The model under review builds one solid part; all positions refer to its coordinate system, in mm. A direction names the side the tool comes from. Give positions to 0.01 mm unless a question says otherwise; leave off trailing zeros. Order: outer loops, then holes, each group sorted by start corner. A loop starts at its lowest first (then second) coordinate and runs counter-clockwise, first axis right, second up. Notation, with made-up numbers: (56, 1) -> (73, 1) arc R12 ccw to (73, 6) -> close; hole circle Ø11 at (-39.5, 36). An arc over 180 degrees is marked (long way). Use one line per item in the form item = value.
```python
from build123d import *

# Parameters (mm, degrees)
SKETCH1_W           = 120
SKETCH1_H           = 75
BOSS_EXTRUDE1_DEPTH = 3
CHAMFER1_SIZE       = 6
SKETCH2_W           = 109.5
SKETCH2_H           = 64.5
BOSS_EXTRUDE2_DEPTH = 2
CHAMFER2_SIZE       = 7
SKETCH3_R           = 1.5
CUT_EXTRUDE1_DEPTH  = 5
SKETCH4_W           = 5.25
SKETCH4_H           = 9.5
SKETCH4_H_2         = 14.5
BOSS_EXTRUDE3_DEPTH = 5


with BuildPart() as part:
    # Sketch1 → Boss-Extrude1 (new body)
    with BuildSketch(Plane(origin=(0, 0, 0), x_dir=(1, 0, 0), z_dir=(0, 1, 0))):
        Rectangle(SKETCH1_W, SKETCH1_H)
    extrude(amount=BOSS_EXTRUDE1_DEPTH)

    # Chamfer1
    chamfer1_edges = [part.edges().sort_by_distance(p)[0] for p in [
        (60, 1.5, 37.5),
        (-60, 1.5, 37.5),
        (-60, 1.5, -37.5),
        (60, 1.5, -37.5),
    ]]
    chamfer(chamfer1_edges, length=CHAMFER1_SIZE)

    # Sketch2 → Boss-Extrude2 (add)
    with BuildSketch(Plane(origin=(0, 3, 0), x_dir=(1, 0, 0), z_dir=(0, 1, 0))):
        Rectangle(SKETCH2_W, SKETCH2_H)
    extrude(amount=BOSS_EXTRUDE2_DEPTH)

    # Chamfer2
    chamfer2_edges = [part.edges().sort_by_distance(p)[0] for p in [
        (54.75, 4, 32.25),
        (54.75, 4, -32.25),
        (-54.75, 4, -32.25),
        (-54.75, 4, 32.25),
    ]]
    chamfer(chamfer2_edges, length=CHAMFER2_SIZE)

    # Sketch3 → Cut-Extrude1 (cut)
    with BuildSketch(Plane(origin=(0, 3, 0), x_dir=(1, 0, 0), z_dir=(0, 1, 0))):
        with Locations(Location((-54.5, -32, 0), (0, 0, 270))):
            Circle(SKETCH3_R)
        with Locations(Location((-54.5, 32, 0), (0, 0, 270))):
            Circle(SKETCH3_R)
        with Locations(Location((54.5, 32, 0), (0, 0, 270))):
            Circle(SKETCH3_R)
        with Locations(Location((54.5, -32, 0), (0, 0, 270))):
            Circle(SKETCH3_R)
    extrude(amount=-CUT_EXTRUDE1_DEPTH, mode=Mode.SUBTRACT)

    # Sketch4 → Boss-Extrude3 (add)
    with BuildSketch(Plane(origin=(0, 3, 0), x_dir=(1, 0, 0), z_dir=(0, 1, 0))):
        with Locations((57.375, 19.5)):
            Rectangle(SKETCH4_W, SKETCH4_H)
        with Locations((57.375, -12)):
            Rectangle(SKETCH4_W, SKETCH4_H_2)
    extrude(amount=BOSS_EXTRUDE3_DEPTH)


solid = part.part
```
1. The part is to be moulded in two halves that separate along Z. For faces 1 (the face through (57, 5, 4.75)), 2 (the face through (54.75, 6, 12)), 3 (the face through (57, 5, 19.25)), 4 (the face through (53.6, 1.5, 30.8)), say which applies: +Z half, -Z half, draft (parallel to the pull), parting line (faces both ways), or undercut.
Values:
face_1 = undercut
face_2 = draft
face_3 = +Z half
face_4 = undercut
2. Tool access review of faces 5 (the face through (57, 5, -24.25)), 6 (the face through (-1, 5, 0)), 7 (the face through (51, 4, 29)), 8 (the face through (57, 5, -14.75)): name each direction out of +Z, -Z, +X, -X, +Y, -Y from which nothing blocks a thin tool from reaching the whole face with its end or side.
Values:
face_5 = -Z, +X, +Y
face_6 = +Z, -Z, -X, +Y
face_7 = +Z, +X, +Y
face_8 = +X, +Y
3. For pin 1 Ø5 at (x, z) = (43, 21.5) entering from -Y; pin 2 Ø0.6 at (y, z) = (3.5, 22) entering from +X; pin 3 Ø0.6 at (y, z) = (4.5, -7) entering from -X; pin 4 Ø2.5 at (y, z) = (7, -20) entering from -X, all flat-tipped, find the tip position at first contact; note any pin that passes through.
Values:
pin_1 = 0
pin_2 = 54.75
pin_3 = -54.75
pin_4 = 54.75
4. Add section C-C on z = -19.5. Give the boundary of the cut face in (x, y), then the cut area to 3 significant figures.
Values:
outline = (-60, 0) -> (60, 0) -> (60, 8) -> (54.75, 8) -> (54.75, 5) -> (-54.75, 5) -> (-54.75, 3) -> (-60, 3) -> close
area = 605 mm^2
5. Add section A-A on y = 6.5. Give the boundary of the cut face in (x, z), then the cut area to 3 significant figures.
Values:
outline = (54.75, -24.25) -> (60, -24.25) -> (60, -14.75) -> (54.75, -14.75) -> close; (54.75, 4.75) -> (60, 4.75) -> (60, 19.25) -> (54.75, 19.25) -> close
area = 126 mm^2
6. For L1, parallel to X at y = 1.55, z = 32; L2, parallel to X at y = 2.25, z = -31.5; L3, parallel to Y at x = 45, z = 30, list the stretches that pass through material, from the lowest coordinate up.
Values:
L1 = -59.5 to -56, -53 to 53, 56 to 59.5
L2 = -60 to -55.91, -53.09 to 53.09, 55.91 to 60
L3 = 0 to 5
7. Add section B-B on x = 20. Give the boundary of the cut face in (y, z), then the cut area to 3 significant figures.
Values:
outline = (0, -37.5) -> (3, -37.5) -> (3, -32.25) -> (5, -32.25) -> (5, 32.25) -> (3, 32.25) -> (3, 37.5) -> (0, 37.5) -> close
area = 354 mm^2
